from build123d import *

# Parameters (mm, degrees)
SKETCH1_W           = 55.1
SKETCH1_H           = 27.8
BOSS_EXTRUDE1_DEPTH = 3
SKETCH2_R           = 1.175
BOSS_EXTRUDE2_DEPTH = 13.4
SKETCH3_W           = 21.65
SKETCH3_H           = 20.203759547
SKETCH3_W_2         = 17.65
SKETCH3_H_2         = 15.75
CUT_EXTRUDE1_DEPTH  = 35.945278651
SKETCH6_W           = 48.551877831
SKETCH6_H           = 2.091403142
SKETCH6_W_2         = 48.7
SKETCH6_H_2         = 4.58395526
CUT_EXTRUDE2_DEPTH  = 1.4


with BuildPart() as part:
    # Sketch1 → Boss-Extrude1 (new body)
    with BuildSketch(Plane(origin=(0, 0, 0), x_dir=(1, 0, 0), z_dir=(0, 1, 0))):
        Rectangle(SKETCH1_W, SKETCH1_H)
    extrude(amount=BOSS_EXTRUDE1_DEPTH)

    # Sketch2 → Boss-Extrude2 (add)
    with BuildSketch(Plane(origin=(0, 3, 0), x_dir=(1, 0, 0), z_dir=(0, 1, 0))):
        with Locations(Location((-25.525, 11.875, 0), (0, 0, 270))):
            Circle(SKETCH2_R)
        with Locations(Location((-25.525, -11.875, 0), (0, 0, 270))):
            Circle(SKETCH2_R)
        with Locations(Location((25.525, 11.875, 0), (0, 0, 270))):
            Circle(SKETCH2_R)
        with Locations(Location((25.525, -11.875, 0), (0, 0, 270))):
            Circle(SKETCH2_R)
    extrude(amount=BOSS_EXTRUDE2_DEPTH)

    # Sketch3 → Cut-Extrude1 (cut, through all)
    # profile 1 of 2: a face of its own
    with BuildSketch(Plane.XZ):
        with Locations((-12.325, -0.13539581)):
            Rectangle(SKETCH3_W, SKETCH3_H)
        with Locations((-12.325, -0.375)):
            Rectangle(SKETCH3_W_2, SKETCH3_H_2, mode=Mode.SUBTRACT)
    # profile 2 of 2: a face of its own
    with BuildSketch(Plane.XZ):
        with Locations((-12.325, -0.375)):
            Rectangle(SKETCH3_W_2, SKETCH3_H_2)
    extrude(amount=-CUT_EXTRUDE1_DEPTH, mode=Mode.SUBTRACT)

    # Sketch6 → Cut-Extrude2 (cut)
    with BuildSketch(Plane(origin=(0, 3, 0), x_dir=(1, 0, 0), z_dir=(0, 1, 0))):
        with Locations((-0.075938916, -12.854298429)):
            Rectangle(SKETCH6_W, SKETCH6_H)
        with Locations((0, 14.16697763)):
            Rectangle(SKETCH6_W_2, SKETCH6_H_2)
    extrude(amount=-CUT_EXTRUDE2_DEPTH, mode=Mode.SUBTRACT)


solid = part.part
Geometry check sheet. Reference: the model listing, model coordinates, mm. A direction names the side the tool comes from. Give positions to 0.01 mm unless a question says otherwise; leave off trailing zeros. Loops run counter-clockwise (first coordinate to the right, second up) from the corner with the lowest first, then second, coordinate; pieces in that order, holes last. Notation, with made-up numbers: (33.5, -38.75) -> (43.5, -38.75) arc R10 ccw to (43.5, -31.75) -> close; hole circle Ø4 at (-19, -11). An arc over 180 degrees is marked (long way). Answer in a Markdown table with one row per item. Add a question column.
1) Draft check along Z on faces 1 (the face through (-12, 1, 9.966)), 2 (the face through (26, 16.4, 12)), 3 (the face through (0, 1, 13.9)). Enter one of: pulls with the +Z half, pulls with the -Z half, needs draft (parallel to the pull), parting line crosses it, or undercut.
2) Cross-section at D-D on y = 8. Record the boundary of the cut face in (x, z) (3 decimals), and give its area (3 significant figures).
3) Gauge pin test, flat ends, axial feed: P1, Ø12, axis at x = -21.5, z = 7.5, coming from the +Y side; P2, Ø5, axis at x = -0.5, z = 1.5, coming from the +Y side; P3, Ø1.7, axis at x = -2.5, z = 13, coming from the +Y side; P4, Ø1.5, axis at x = 9, y = 2.5, coming from the -Z side (3 decimals). Record the tip position at first contact, or that the pin passes through.
4) Cross-section at B-B on x = -9. Record the boundary of the cut face in (y, z) (3 decimals), and give its area (3 significant figures).
5) Material ranges on probe 1 along Z at (x, y) = (-13, 2) (3 decimals); probe 2 along X at (y, z) = (7, -12); probe 3 along Z at (x, y) = (-3.5, 1.5), recorded low to high. Write a range as from..to.
6) Cross-section at A-A on z = 0.75. Record the boundary of the cut face in (x, y).
7) Set-up check for faces 4 (the face through (-12, 1, -10.237)), 5 (the face through (-26.24, 9.606, -12.807)), 6 (the face through (-24.352, 2, 13)), 7 (the face through (-24.35, 2, -13)), 8 (the face through (26, 16.4, -12)): record each of +Z, -Z, +X, -X, +Y, -Y from which the full face is reachable in a straight line by a thin tool's end or side.
8) Cross-section at C-C on x = 13.5. Record the boundary of the cut face in (y, z) (3 decimals), and give its area (3 significant figures).
Outcome:
| question | item | result |
|---|---|---|
| 1 | face 1 | undercut |
| 1 | face 2 | needs draft |
| 1 | face 3 | pulls with the +Z half |
| 2 | outline | circle Ø2.35 at (-25.525, -11.875); circle Ø2.35 at (-25.525, 11.875); circle Ø2.35 at (25.525, -11.875); circle Ø2.35 at (25.525, 11.875) |
| 2 | area | 17.3 mm^2 |
| 3 | P1 | stops at y = 16.4 |
| 3 | P2 | stops at y = 3 |
| 3 | P3 | stops at y = 1.6 |
| 3 | P4 | stops at z = -11.875 |
| 4 | outline | (0, -13.9) -> (1.6, -13.9) -> (1.6, -11.875) -> (3, -11.875) -> (3, -10.237) -> (0, -10.237) -> close; (0, 9.966) -> (3, 9.966) -> (3, 11.809) -> (1.6, 11.809) -> (1.6, 13.9) -> (0, 13.9) -> close |
| 4 | area | 17.0 mm^2 |
| 5 | probe 1 | z = -11.875..-10.237, 9.966..11.809 |
| 5 | probe 2 | x = -26.69..-24.36, 24.36..26.69 |
| 5 | probe 3 | z = -13.9..-10.24, 9.97..13.9 |
| 6 | outline | (-27.55, 0) -> (-23.15, 0) -> (-23.15, 3) -> (-27.55, 3) -> close; (-1.5, 0) -> (27.55, 0) -> (27.55, 3) -> (-1.5, 3) -> close |
| 7 | face 4 | +Y, -Y |
| 7 | face 5 | +Y |
| 7 | face 6 | +Z, +Y |
| 7 | face 7 | -Z, +Y |
| 7 | face 8 | +Z, -Z, +X, -X, +Y |
| 8 | outline | (0, -13.9) -> (1.6, -13.9) -> (1.6, -11.875) -> (3, -11.875) -> (3, 11.809) -> (1.6, 11.809) -> (1.6, 13.9) -> (0, 13.9) -> close |
| 8 | area | 77.6 mm^2 |
